```python
from build123d import *

# Parameters (mm, degrees)
F0_R     = 8.128
F1_DEPTH = 12.7
F5_DEPTH = 12.701


# Not quite as in the source:
# - ends of sketch curves that miss each other by under 0.0002 mm in the source are joined


with BuildPart() as f1:
    # F0 (on Front) → F1 (new body)
    with BuildSketch(Plane.XZ):
        with BuildLine():
            Line((-5.0256186, 25.460071), (-14.7940014, 8.54075))
            ThreePointArc((-14.7940014, 8.54075), (-14.7940038016, -8.5407495378), (-0.0009906, -17.0815))
            ThreePointArc((-0.0009906, -17.0815), (22.5453798959, 2.8340109101), (4.2845187845, 26.7402328229))
            ThreePointArc((4.2845187845, 26.7402328229), (0.7827449758, 27.0701370063), (-2.7322519698, 26.9433993832))
            ThreePointArc((-2.7322519698, 26.9433993832), (-4.0577155326, 26.4781440431), (-5.0256186, 25.460071))
        make_face()
        with Locations((-0.0009906, 0)):
            Circle(F0_R, mode=Mode.SUBTRACT)
    extrude(amount=-F1_DEPTH)

    # F2 (on Top) → F3 (revolve, cut)
    with BuildSketch(Plane.XY):
        Polygon((1.778, 0), (8.128, 0), (12.4623477688, 12.954), (8.128, 12.954), (1.778, 12.954), align=None)
    revolve(axis=Axis((-0.0009906, 0, 0), (0, -1, 0)), mode=Mode.SUBTRACT)

    # F4 (on face) → F5 (cut, through all)
    with BuildSketch(Plane.XZ):
        with BuildLine():
            Line((-1.5875, 13.97), (-1.5875, 3.0828800518))
            Line((-1.5875, 3.0828800518), (1.5875, 3.0828800518))
            Line((1.5875, 3.0828800518), (1.5875, 13.97))
            ThreePointArc((1.5875, 13.97), (0, 15.5575), (-1.5875, 13.97))
        make_face()
    extrude(amount=-F5_DEPTH, mode=Mode.SUBTRACT)


solid = f1.part
```
Check sheet for the modelled part. Datum: model origin and axes. Units: mm. A direction names the side the tool comes from. Give positions to 0.01 mm unless a question says otherwise; leave off trailing zeros. Loops run counter-clockwise (first coordinate to the right, second up) from the corner with the lowest first, then second, coordinate; pieces in that order, holes last. Notation, with made-up numbers: M 40.25,52 L 68.25,52 A27 cw 68.25,87 Z; hole C 22.25,85.25 d6. An arc over 180 degrees is marked long. Answer as CSV lines item,"result".
Item 1: Draft check along X on faces 3 (the face through (0.83, 6.26, 27.07)), 4 (the face through (0.035, 6.261, 15.557)), 5 (the face through (-4.04, 6.26, 26.49)). Enter one of: pulls with the +X half, pulls with the -X half, needs draft (parallel to the pull), parting line crosses it, or undercut.
Reply:
face 3,"parting line crosses it"
face 4,"undercut"
face 5,"pulls with the -X half"
Item 2: Set-up check for faces 1 (the face through (-1.588, 5, 12)), 2 (the face through (11, 12.7, 10)): record each of +Z, -Z, +X, -X, +Y, -Y from which the full face is reachable in a straight line by a thin tool's end or side.
Reply:
face 1,"+Y, -Y"
face 2,"+Z, -Z, +X, -X, +Y"
Item 3: Sectioned sample at C-C, the plane y = 3.75. Enter the section's corners in (x, z) (1 decimal), then the cut area to 3 significant figures.
Reply:
outline,"M -14.8,8.5 A17.1 ccw 0,-17.1 A22.1 ccw 4.3,26.7 A27.1 ccw -2.7,26.9 A3 ccw -5,25.5 Z; hole M -1.6,9.2 A9.4 ccw long 1.6,9.2 L 1.6,14 A1.6 ccw -1.6,14 Z"
area,"1,040 mm^2"
Item 4: Sectioned sample at D-D, the plane x = 14. Enter the section's corners in (y, z), then the cut area to 3 significant figures.
Reply:
outline,"M 0,-12.54 L 12.7,-12.54 L 12.7,22.5 L 0,22.5 Z"
area,"445 mm^2"
Item 5: Scan lines: L1, parallel to X at y = 0.5, z = -1.5; L2, parallel to X at y = 7, z = -1; L3, parallel to Z at x = -0.5, y = 8.25. Record each from-to range of solid material in increasing order.
Reply:
L1,"-17.02 to -8.16, 8.16 to 21.68"
L2,"-17.05 to -10.42, 10.42 to 21.82"
L3,"-17.07 to -10.88, 15.48 to 27.08"
Item 6: Sectioned sample at B-B, the plane y = 1.25. Enter the section's corners in (x, z) (1 decimal).
Reply:
outline,"M -14.8,8.5 A17.1 ccw 0,-17.1 A22.1 ccw 4.3,26.7 A27.1 ccw -2.7,26.9 A3 ccw -5,25.5 Z; hole M -1.6,8.4 A8.5 ccw long 1.6,8.4 L 1.6,14 A1.6 ccw -1.6,14 Z"
Item 7: Depth check by flat-ended pin: pin 1 Ø4 at (y, z) = (4, -9) entering from -X; pin 2 Ø1.5 at (x, y) = (3.5, 5) entering from +Z; pin 3 Ø4 at (x, y) = (16, 6) entering from -Z. Enter the tip coordinate at first touch or a pass-through.
Reply:
pin 1,"x = -15.58"
pin 2,"z = 26.94"
pin 3,"z = -12.54"
Item 8: Sectioned sample at A-A, the plane z = 0. Enter the section's corners in (x, y).
Reply:
outline,"M -17.08,0 L -8.13,0 L -12.38,12.7 L -17.08,12.7 Z; M 8.13,0 L 22.08,0 L 22.08,12.7 L 12.38,12.7 Z"
